Here's the drawing with two shaded views (mm, measured from the low corner). I have some questions. Give positions to 0.01 mm unless a question says otherwise; leave off trailing zeros. Write each loop counter-clockwise with the first axis right and the second up, starting at its lowest first coordinate (ties: lowest second). Pieces come first, ordered by that corner, then holes.
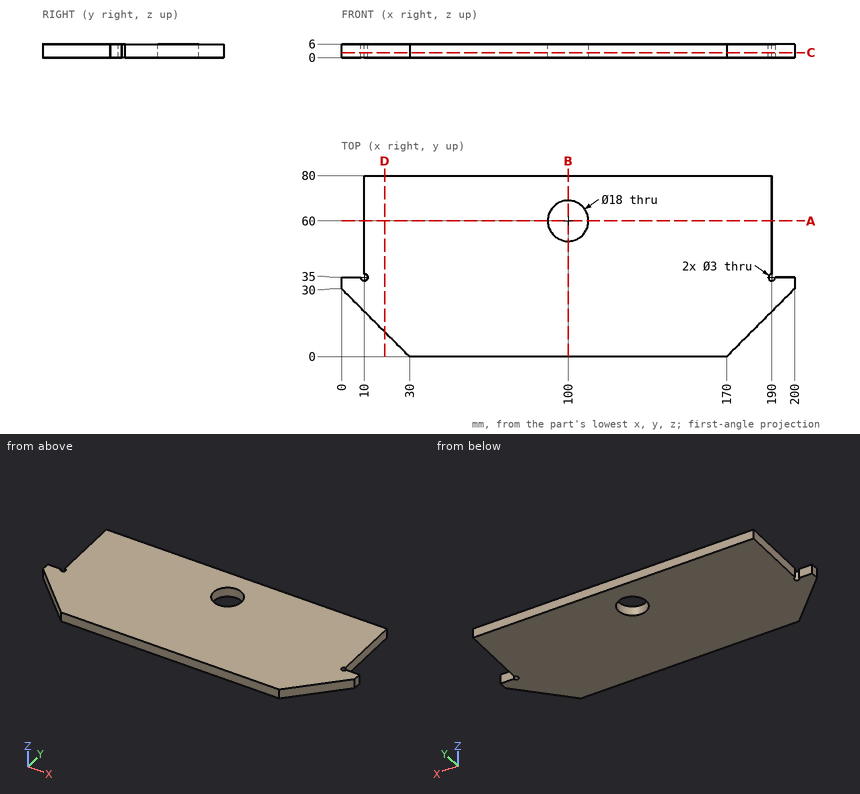
(1) Imagine slicing it at D-D, the plane x = 19. Write out the boundary of the cut face in (y, z).
Returned:
outline: (11, 0) - (80, 0) - (80, 6) - (11, 6) - close
(2) If I drill on L1, parallel to X at y = 60, z = 4.25; L2, parallel to X at y = 67, z = 3.3; L3, parallel to Y at x = 100, z = 3.1, over which ranges is the centre line in solid material (lowest first)?
Returned:
L1: x = 10 to 91, 109 to 190
L2: x = 10 to 94.34, 105.66 to 190
L3: y = 0 to 51, 69 to 80
(3) Imagine slicing it at A-A, the plane y = 60. Write out the boundary of the cut face in (x, z), plus the area to 3 significant figures.
Returned:
outline: (10, 0) - (91, 0) - (91, 6) - (10, 6) - close; (109, 0) - (190, 0) - (190, 6) - (109, 6) - close
area: 972 mm2
(4) Imagine slicing it at C-C, the plane z = 2.15. Write out the boundary of the cut face in (x, y).
Returned:
outline: (0, 30) - (30, 0) - (170, 0) - (200, 30) - (200, 35) - (191.5, 35) arc R1.5 cw (long way) to (190, 36.5) - (190, 80) - (10, 80) - (10, 36.5) arc R1.5 cw (long way) to (8.5, 35) - (0, 35) - close; hole circle Ø18 at (100, 60)
(5) Will these pins go through, and if not, where does the flat tip stop? P1, Ø3, axis at x = 6, z = 4, coming from the +Y side; P2, Ø3, axis at y = 25.5, z = 1.5, coming from the +X side; P3, Ø1.8, axis at y = 68, z = 3, coming from the -X side.
Returned:
P1: stops at y = 35
P2: stops at x = 197
P3: stops at x = 10
(6) Imagine slicing it at B-B, the plane x = 100. Write out the boundary of the cut face in (y, z).
Returned:
outline: (0, 0) - (51, 0) - (51, 6) - (0, 6) - close; (69, 0) - (80, 0) - (80, 6) - (69, 6) - close
